For this review, use the dimensioned drawing (mm, ordinates from the lowest corner) and the shaded views. A direction names the side the tool comes from. Coordinates: 2 decimals unless noted, no trailing zeros. Loops run counter-clockwise (first coordinate to the right, second up) from the corner with the lowest first, then second, coordinate; pieces in that order, holes last. Notation, with made-up numbers: (57, 67) - (61, 67) arc R11 ccw to (61, 79) - close; hole circle Ø9 at (69.25, 11). An arc over 180 degrees is marked (long way). Use one line per item in the form item = value. Start each with the question number.
(1) Add section C-C (z = 61). State the section outline as (x, y) points.
(2) Add section B-B (x = 11). State the section outline as (y, z) points.
(3) Clearance check with flat-ended pins moving along their axes: pin 1 Ø14.5 at (x, z) = (111, 61) entering from -Y; pin 2 Ø11.5 at (x, z) = (111, 11) entering from +Y; pin 3 Ø8 at (x, z) = (88, 43.5) entering from +Y; pin 4 Ø3 at (y, z) = (36, 58) entering from -X. State where each tip first meets the part, or that it passes through.
(4) Tool access review of the marked faces 1, 2 and 3: name each direction out of +Z, -Z, +X, -X, +Y, -Y from which nothing blocks a thin tool from reaching the whole face with its end or side.
(5) Add section D-D (x = 61). State the section outline as (y, z) points, plus the area to 3 significant figures.
(6) Add section A-A (y = 52). State the section outline as (x, z) points, plus the area to 3 significant figures.
(7) The part is to be moulded in two halves that separate along X. For the marked faces 4, 5 and 6, say which applies: pulls with the +X half, pulls with the -X half, needs draft (parallel to the pull), parting line crosses it, or undercut.
(8) For L1, parallel to Z at x = 111, y = 19.5; L2, parallel to X at y = 52, z = 39.5; L3, parallel to X at y = 52, z = 57.5, list the stretches that pass through material, from the lowest coordinate up.
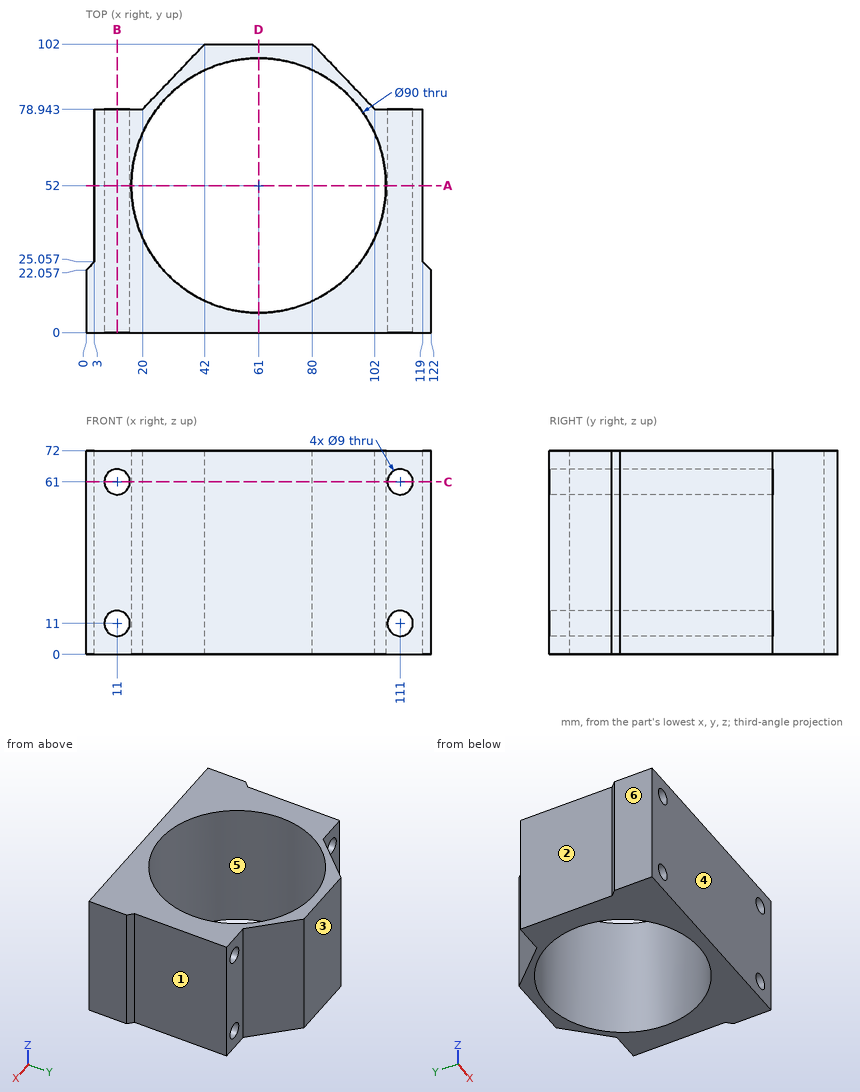
Computed values:
q1.outline = (0, 0) - (6.5, 0) - (6.5, 78.94) - (3, 78.94) - (3, 25.06) - (0, 22.06) - close; (15.5, 0) - (106.5, 0) - (106.5, 78.94) - (102, 78.94) - (80, 102) - (42, 102) - (20, 78.94) - (15.5, 78.94) - close; (115.5, 0) - (122, 0) - (122, 22.06) - (119, 25.06) - (119, 78.94) - (115.5, 78.94) - close; hole circle Ø90 at (61, 52)
q2.outline = (0, 0) - (78.94, 0) - (78.94, 6.5) - (0, 6.5) - close; (0, 15.5) - (78.94, 15.5) - (78.94, 56.5) - (0, 56.5) - close; (0, 65.5) - (78.94, 65.5) - (78.94, 72) - (0, 72) - close
q3.pin_1 = 0
q3.pin_2 = 78.94
q3.pin_3 = 97.81
q3.pin_4 = 3
q4.face_1 = +Z, -Z, +X, +Y
q4.face_2 = +Z, -Z, -X, +Y
q4.face_3 = +Z, -Z, +X, -X, +Y
q5.outline = (0, 0) - (7, 0) - (7, 72) - (0, 72) - close; (97, 0) - (102, 0) - (102, 72) - (97, 72) - close
q5.area = 864 mm^2
q6.outline = (3, 0) - (16, 0) - (16, 72) - (3, 72) - close; (106, 0) - (119, 0) - (119, 72) - (106, 72) - close; hole circle Ø9 at (11, 11); hole circle Ø9 at (11, 61); hole circle Ø9 at (111, 11); hole circle Ø9 at (111, 61)
q6.area = 1,620 mm^2
q7.face_4 = needs draft
q7.face_5 = undercut
q7.face_6 = pulls with the -X half
q8.L1 = 0 to 6.5, 15.5 to 56.5, 65.5 to 72
q8.L2 = 3 to 16, 106 to 119
q8.L3 = 3 to 8.17, 13.83 to 16, 106 to 108.17, 113.83 to 119
